Geometry check sheet. Reference: the model listing, model coordinates, mm. Face numbers are marked on the shaded views. A direction names the side the tool comes from. Give positions to 0.01 mm unless a question says otherwise; leave off trailing zeros. Order: outer loops, then holes, each group sorted by start corner. A loop starts at its lowest first (then second) coordinate and runs counter-clockwise, first axis right, second up. Notation, with made-up numbers: M 4.5,1 L 13.5,1 A6 cw 13.5,6 Z; hole C 32,81 d8. An arc over 180 degrees is marked long. Answer as CSV lines item,"result".
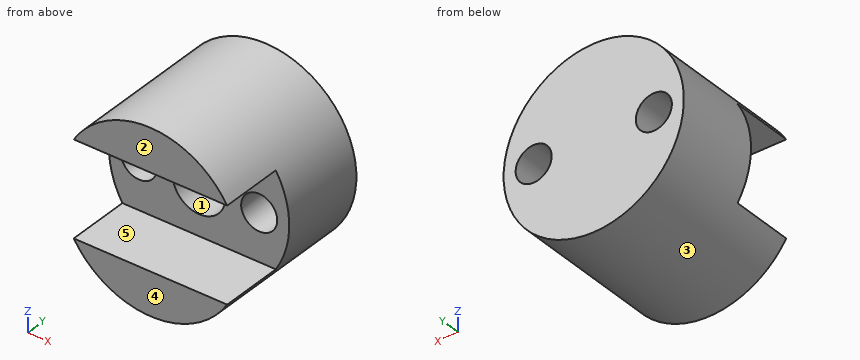
from build123d import *

# Parameters (mm, degrees)
SKETCH_1_R          = 6
EXTRUDE_1_DEPTH     = 10
CUT_EXTRUDE_1_DEPTH = 4.2
SKETCH_3_R          = 1.75
CUT_EXTRUDE_2_DEPTH = 5.5
SKETCH_4_R          = 1.2
CUT_EXTRUDE_3_DEPTH = 5.8


with BuildPart() as part:
    # Эскиз1 → Бобышка-Вытянуть1 (new body)
    with BuildSketch(Plane(origin=(0, 0, 0), x_dir=(1, 0, 0), z_dir=(0, 1, 0))):
        with Locations(Location((0, 0, 0), (0, 0, 270))):
            Circle(SKETCH_1_R)
    extrude(amount=EXTRUDE_1_DEPTH)

    # Эскиз2 → Вырез-Вытянуть1 (cut)
    with BuildSketch(Plane.XZ):
        with BuildLine():
            Line((-5.106613359, 3.15), (5.106613359, 3.15))
            ThreePointArc((5.106613359, 3.15), (6, 0), (5.106613359, -3.15))
            Line((5.106613359, -3.15), (-5.106613359, -3.15))
            ThreePointArc((-5.106613359, -3.15), (-6, 0), (-5.106613359, 3.15))
        make_face()
    extrude(amount=-CUT_EXTRUDE_1_DEPTH, mode=Mode.SUBTRACT)

    # Эскиз3 → Вырез-Вытянуть2 (cut)
    with BuildSketch(Plane.XZ.offset(-4.2)):
        with Locations(Location((0, 0, 0), (0, 0, 270))):
            Circle(SKETCH_3_R)
    extrude(amount=-CUT_EXTRUDE_2_DEPTH, mode=Mode.SUBTRACT)

    # Эскиз4 → Вырез-Вытянуть3 (cut)
    with BuildSketch(Plane.XZ.offset(-4.2)):
        with Locations(Location((-4, 0, 0), (0, 0, 270))):
            Circle(SKETCH_4_R)
        with Locations(Location((4, 0, 0), (0, 0, 90))):
            Circle(SKETCH_4_R)
    extrude(amount=-CUT_EXTRUDE_3_DEPTH, mode=Mode.SUBTRACT)


solid = part.part
(1) Section check D-D on y = 1.5. Enter the section's corners in (x, z).
The answers:
outline,"M -5.11,-3.15 A6 ccw 5.11,-3.15 Z; M -5.11,3.15 L 5.11,3.15 A6 ccw Z"
(2) Section check C-C on y = 7.5. Enter the section's corners in (x, z).
The answers:
outline,"C 0,0 d12; hole C -4,0 d2.4; hole C 0,0 d3.5; hole C 4,0 d2.4"
(3) Section check B-B on x = 3.5. Enter the section's corners in (y, z).
The answers:
outline,"M 0,-4.87 L 10,-4.87 L 10,-1.09 L 4.2,-1.09 L 4.2,-3.15 L 0,-3.15 Z; M 0,3.15 L 4.2,3.15 L 4.2,1.09 L 10,1.09 L 10,4.87 L 0,4.87 Z"
(4) Draft check along X on the marked faces 1, 2 and 3. Enter one of: +X half, -X half, draft (parallel to the pull), parting line (faces both ways), or undercut.
The answers:
face 1,"undercut"
face 2,"draft"
face 3,"parting line"
(5) Section check A-A on z = 0. Enter the section's corners in (x, y).
The answers:
outline,"M -6,4.2 L -5.2,4.2 L -5.2,10 L -6,10 Z; M -2.8,4.2 L -1.75,4.2 L -1.75,9.7 L 1.75,9.7 L 1.75,4.2 L 2.8,4.2 L 2.8,10 L -2.8,10 Z; M 5.2,4.2 L 6,4.2 L 6,10 L 5.2,10 Z"
(6) Tool access check on the marked faces 4 and 5. Record the directions out of +Z, -Z, +X, -X, +Y, -Y that give a thin tool (end or side, any length) a straight path to the whole face; none if there is none.
The answers:
face 4,"+Z, -Z, +X, -X, -Y"
face 5,"+X, -X, -Y"
(7) Material ranges on line 1 (X direction, y = 7.3, z = 0); line 2 (X direction, y = 6.25, z = -0.5); line 3 (Z direction, x = -4.5, y = 3.5), recorded low to high.
The answers:
line 1,"x = -6 to -5.2, -2.8 to -1.75, 1.75 to 2.8, 5.2 to 6"
line 2,"x = -5.98 to -5.09, -2.91 to -1.68, 1.68 to 2.91, 5.09 to 5.98"
line 3,"z = -3.97 to -3.15, 3.15 to 3.97"
(8) Gauge pin test, flat ends, axial feed: P1, Ø4, axis at x = 0, z = 0, coming from the -Y side; P2, Ø4.5, axis at x = 2.5, y = 2.5, coming from the +Z side; P3, Ø1.4, axis at x = 4, z = 0, coming from the +Y side; P4, Ø1.5, axis at y = 3, z = 4.5, coming from the -X side. Record the tip position at first contact, or that the pin passes through.
The answers:
P1,"stops at y = 4.2"
P2,"stops at z = 5.99"
P3,"passes through"
P4,"stops at x = -4.68"
